CAD build for the part. Positions are in the model's coordinates, mm. Face numbers are marked on the shaded views. A direction names the side the tool comes from. Coordinates: 2 decimals unless noted, no trailing zeros. Loops run counter-clockwise (first coordinate to the right, second up) from the corner with the lowest first, then second, coordinate; pieces in that order, holes last.
1) Saw through at A-A, the plane y = 0. Write the cut outline in (x, z), and give its area (3 significant figures).
2) Pin check, flat tips, straight feed: pin 1 Ø1.9 at (x, y) = (0, 1.5) entering from +Z; pin 2 Ø2 at (x, z) = (-2.5, 2) entering from -Y; pin 3 Ø2 at (x, z) = (0.5, 3) entering from -Y; pin 4 Ø4 at (x, y) = (0, 0) entering from -Z. Stop position of each tip, or through.
3) Two-plate mould, pull along X, no slides. Class the marked faces 1, 2 and 3: +X half, -X half, draft (parallel to the pull), parting line (faces both ways), or undercut.
4) Saw through at C-C, the plane z = 0.75. Write the cut outline in (x, y) (1 decimal).
5) Which spindle directions (+Z, -Z, +X, -X, +Y, -Y) get a long thin tool onto all of the face, cutting with end or side? Do the marked faces 4 and 5. Say none if no direction does.
6) Wall check: line 1 along X through (y, z) = (0.25, 4.05); line 2 along Z through (x, y) = (0.75, 2.75); line 3 along X through (y, z) = (-1, 2.35). Give the ranges that are in metal, low to high.
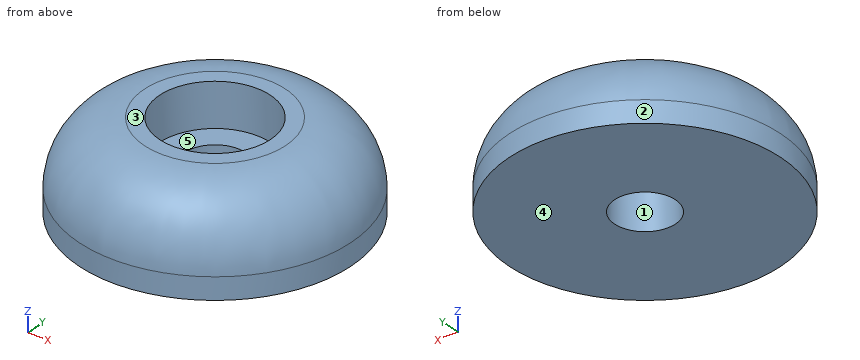
Autodesk Inventor part; units mm, degrees
ref_plane "YZ Plane" through (0, 0, 0) normal (1, 0, 0) x (0, 1, 0)
ref_plane "XZ Plane" through (0, 0, 0) normal (0, 1, 0) x (-1, 0, 0)
ref_plane "XY Plane" through (0, 0, 0) normal (0, 0, 1) x (1, 0, 0)
sketch "Sketch1" plane through (0, 0, 0) normal (0, 0, 1) x (1, 0, 0)
  circle A0 centre (0, 0) radius 1.778
  circle A1 centre (0, 0) radius 7.9375
  dimension "d0" = 3.556
  dimension "d1" = 15.875
extrude "Extrusion1" add sketch "Sketch1" along normal blind 5.08
sketch "Sketch2" plane through (0, 0, 5.08) normal (0, 0, 1) x (1, 0, 0)
  circle A0 centre (0, 0) radius 1.778
  circle A1 centre (0, 0) radius 3.2385
  dimension "d4" = 6.477
extrude "Extrusion2" cut sketch "Sketch2" against normal blind 2.54
fillet "Fillet1" radius 3.81 1 edges at (-7.9375, 0, 5.08)
properties part number "HANDLE WASHER"
Data:
1. outline: (-7.94, 0) - (-1.78, 0) - (-1.78, 2.54) - (-3.24, 2.54) - (-3.24, 5.08) - (-4.13, 5.08) arc R3.81 ccw to (-7.94, 1.27) - close; (1.78, 0) - (7.94, 0) - (7.94, 1.27) arc R3.81 ccw to (4.13, 5.08) - (3.24, 5.08) - (3.24, 2.54) - (1.78, 2.54) - close
1. area: 48.9 mm2
2. pin 1: stops at z = 2.54
2. pin 2: stops at y = -7.76
2. pin 3: stops at y = -7.86
2. pin 4: stops at z = 0
3. face 1: undercut
3. face 2: parting line
3. face 3: draft
4. outline: circle Ø15.9 at (0, 0); hole circle Ø3.6 at (0, 0)
5. face 4: -Z, +X, -X, +Y, -Y
5. face 5: +Z
6. line 1: x = -6.73 to -3.23, 3.23 to 6.73
6. line 2: z = 0 to 2.54
6. line 3: x = -7.72 to -1.47, 1.47 to 7.72
